Verification items for the finished model (mm, model axes). Face numbers are marked on the shaded views. A direction names the side the tool comes from. Coordinates: 2 decimals unless noted, no trailing zeros. Order: outer loops, then holes, each group sorted by start corner. A loop starts at its lowest first (then second) coordinate and runs counter-clockwise, first axis right, second up. Notation, with made-up numbers: (-36.5, -36.5) -> (9.5, -36.5) arc R26 ccw to (9.5, -18.5) -> close; hole circle Ø3 at (-9, -30). An arc over 180 degrees is marked (long way). Write each question's results on one line, items separated by ' | '. Start each with the question number.
(1) Draft check along X on the marked faces 1, 2, 3 and 4. Enter one of: +X half, -X half, draft (parallel to the pull), parting line (faces both ways), or undercut.
(2) Cross-section at D-D on y = 15. Enter the section's corners in (x, z), and give its area (3 significant figures).
(3) Cross-section at A-A on y = 3. Enter the section's corners in (x, z) (3 decimals).
(4) Go/stop test with flat-tipped pins: pin 1 (3.5 mm diameter, centred on x = 8.5, y = 12.5, fed in from +Z); pin 2 (4 mm diameter, centred on x = 3.5, y = 15, fed in from -Z). Record where each tip stops, or that it passes through.
(5) Cross-section at B-B on x = 13.5. Enter the section's corners in (y, z) (3 decimals), and give its area (3 significant figures).
(6) Cross-section at C-C on z = 0.8. Enter the section's corners in (x, y) (3 decimals), and give its area (3 significant figures).
(7) Set-up check for the marked faces 5 and 6: record each of +Z, -Z, +X, -X, +Y, -Y from which the full face is reachable in a straight line by a thin tool's end or side.
(8) Thickness scan on probe 1 along Y at (x, z) = (2.7, 1.55) (3 decimals); probe 2 along Z at (x, y) = (8.5, 15.5); probe 3 along X at (y, z) = (4.25, 0.95). Record the ranges inside material, lowest first. Write a range as [from, to].
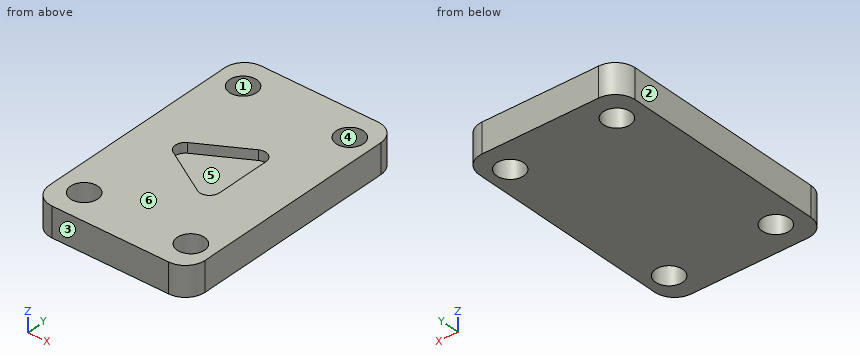
```python
from build123d import *

# Parameters (mm, degrees)
F0_W      = 15.8
F0_H      = 25
F1_DEPTH  = 3
F3_R      = 1.375
F4_R      = 1.375
F7_DEPTH  = 5
F5_R      = 1.375
F8_DEPTH  = 5
F6_R      = 1.375
F9_DEPTH  = 5
F10_R     = 2
F12_DEPTH = 1
F13_R     = 1


with BuildPart() as f1:
    # F0 (on Top) → F1 (new body)
    with BuildSketch(Plane.XY):
        with Locations((7.9, 12.5)):
            Rectangle(F0_W, F0_H)
    extrude(amount=F1_DEPTH)

    # F3 (on face) + F4 (on face) → F7 (cut)
    with BuildSketch(Plane.XY.offset(3)):
        with Locations((13.5, 3)):
            Circle(F3_R)
    with BuildSketch(Plane.XY.offset(3)):
        with Locations((2.7, 3)):
            Circle(F4_R)
    extrude(amount=-F7_DEPTH, mode=Mode.SUBTRACT)

    # F5 (on face) → F8 (cut)
    with BuildSketch(Plane.XY.offset(3)):
        with Locations((2.7, 22)):
            Circle(F5_R)
    extrude(amount=-F8_DEPTH, mode=Mode.SUBTRACT)

    # F6 (on face) → F9 (cut)
    with BuildSketch(Plane.XY.offset(3)):
        with Locations((13.5, 22)):
            Circle(F6_R)
    extrude(amount=-F9_DEPTH, mode=Mode.SUBTRACT)

    # F10
    f10_edges = [f1.edges().sort_by_distance(p)[0] for p in [
        (15.8, 25, 1.5),
        (15.8, 0, 1.5),
        (0, 0, 1.5),
        (0, 25, 1.5),
    ]]
    fillet(f10_edges, radius=F10_R)

    # F11 (on face) → F12 (cut)
    with BuildSketch(Plane.XY.offset(3)):
        Polygon((10.7, 17.003332), (2.9, 12.5), (10.7, 7.996668), align=None)
    extrude(amount=-F12_DEPTH, mode=Mode.SUBTRACT)

    # F13
    f13_edges = [f1.edges().sort_by_distance(p)[0] for p in [
        (2.9, 12.5, 2.5),
        (10.7, 17.003332, 2.5),
        (10.7, 7.996668, 2.5),
    ]]
    fillet(f13_edges, radius=F13_R)


solid = f1.part
```
Results are:
1) face 1: undercut | face 2: -X half | face 3: draft | face 4: undercut
2) outline: (0, 0) -> (15.8, 0) -> (15.8, 3) -> (10.7, 3) -> (10.7, 2) -> (7.23, 2) -> (7.23, 3) -> (0, 3) -> close | area: 43.9 mm2
3) outline: (0, 0) -> (1.325, 0) -> (1.325, 3) -> (0, 3) -> close; (4.075, 0) -> (12.125, 0) -> (12.125, 3) -> (4.075, 3) -> close; (14.875, 0) -> (15.8, 0) -> (15.8, 3) -> (14.875, 3) -> close
4) pin 1: stops at z = 2 | pin 2: stops at z = 0
5) outline: (0, 0) -> (1.625, 0) -> (1.625, 3) -> (0, 3) -> close; (4.375, 0) -> (20.625, 0) -> (20.625, 3) -> (4.375, 3) -> close; (23.375, 0) -> (25, 0) -> (25, 3) -> (23.375, 3) -> close | area: 58.5 mm2
6) outline: (0, 2) arc R2 ccw to (2, 0) -> (13.8, 0) arc R2 ccw to (15.8, 2) -> (15.8, 23) arc R2 ccw to (13.8, 25) -> (2, 25) arc R2 ccw to (0, 23) -> close; hole circle Ø2.75 at (2.7, 3); hole circle Ø2.75 at (2.7, 22); hole circle Ø2.75 at (13.5, 3); hole circle Ø2.75 at (13.5, 22) | area: 368 mm2
7) face 5: +Z | face 6: +Z, +X, -X, +Y, -Y
8) probe 1: y = [0, 1.625], [4.375, 20.625], [23.375, 25] | probe 2: z = [0, 2] | probe 3: x = [0, 2.13], [3.27, 12.93], [14.07, 15.8]
